Print and shaded views of the part. All mm, measured from the part's lowest x, y and z. A direction names the side the tool comes from. Round coordinates to 2 decimals unless told otherwise and drop trailing zeros. Write each loop counter-clockwise with the first axis right and the second up, starting at its lowest first coordinate (ties: lowest second). Pieces come first, ordered by that corner, then holes.
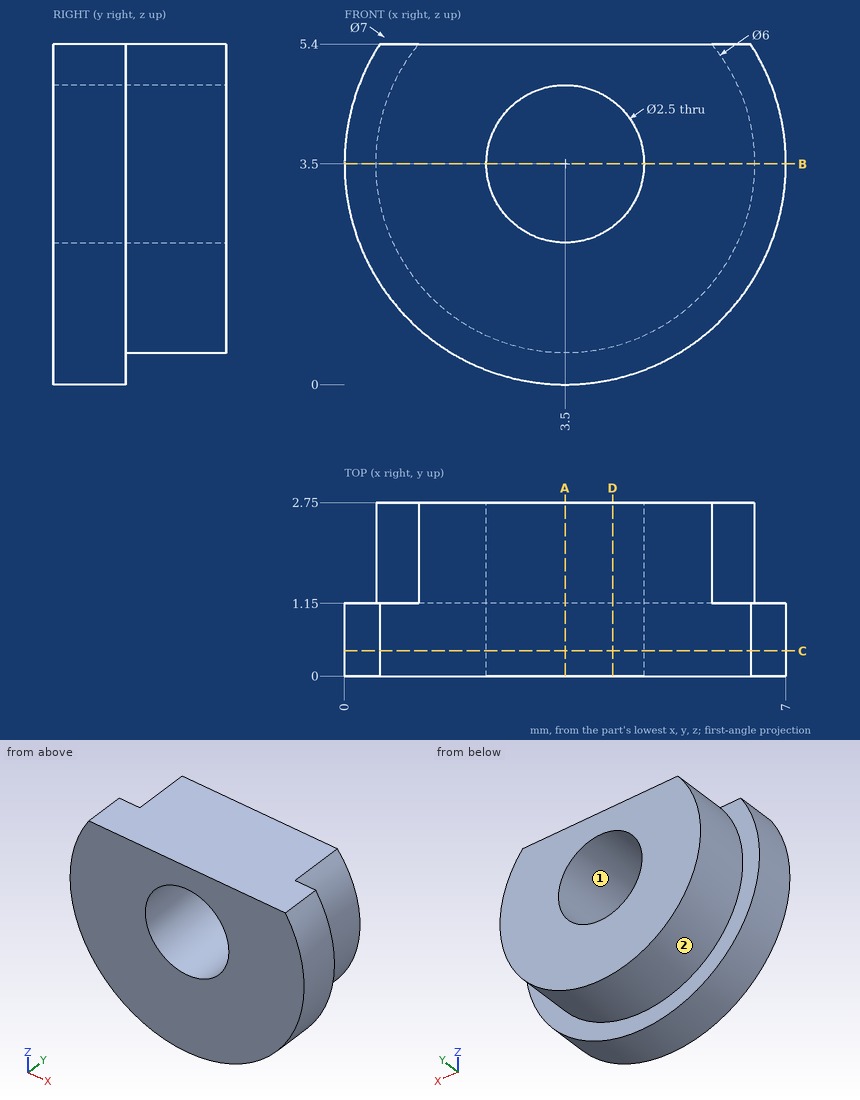
1) Slice it at B-B (z = 3.5). Write the cut outline in (x, y).
Results:
outline: (0, 0) - (2.25, 0) - (2.25, 2.75) - (0.5, 2.75) - (0.5, 1.15) - (0, 1.15) - close; (4.75, 0) - (7, 0) - (7, 1.15) - (6.5, 1.15) - (6.5, 2.75) - (4.75, 2.75) - close
2) Pin check, flat tip, straight feed: pin 1 Ø2 at (x, z) = (3.5, 3.5) entering from +Y. Stop position of the tip, or through.
Results:
pin 1: passes through
3) Slice it at C-C (y = 0.4). Write the cut outline in (x, z), plus the area to 3 significant figures.
Results:
outline: (0.56, 5.4) arc R3.5 ccw (long way) to (6.44, 5.4) - close; hole circle Ø2.5 at (3.5, 3.5)
area: 26.9 mm2
4) Which spindle directions (+Z, -Z, +X, -X, +Y, -Y) get a long thin tool onto all of the face, cutting with end or side? Do the marked faces 1 and 2. Say none if no direction does.
Results:
face 1: +Y, -Y
face 2: +Y
5) Wall check: L1, parallel to X at y = 1.05, z = 3.5; L2, parallel to Z at x = 3.5, y = 1.65; L3, parallel to X at y = 2.05, z = 3.5. Give the ranges that are in metal, low to high.
Results:
L1: x = 0 to 2.25, 4.75 to 7
L2: z = 0.5 to 2.25, 4.75 to 5.4
L3: x = 0.5 to 2.25, 4.75 to 6.5
6) Slice it at D-D (x = 4.25). Write the cut outline in (y, z), plus the area to 3 significant figures.
Results:
outline: (0, 0.08) - (1.15, 0.08) - (1.15, 0.6) - (2.75, 0.6) - (2.75, 2.5) - (0, 2.5) - close; (0, 4.5) - (2.75, 4.5) - (2.75, 5.4) - (0, 5.4) - close
area: 8.30 mm2
7) Slice it at A-A (x = 3.5). Write the cut outline in (y, z).
Results:
outline: (0, 0) - (1.15, 0) - (1.15, 0.5) - (2.75, 0.5) - (2.75, 2.25) - (0, 2.25) - close; (0, 4.75) - (2.75, 4.75) - (2.75, 5.4) - (0, 5.4) - close
